Could you check a few things on this model? Use its own coordinates, in mm. Give positions to 0.01 mm unless a question says otherwise; leave off trailing zeros. Loops run counter-clockwise (first coordinate to the right, second up) from the corner with the lowest first, then second, coordinate; pieces in that order, holes last. Notation, with made-up numbers: (-34.5, 2) - (-24.5, 2) arc R31 ccw to (-24.5, 38) - close; hole circle Ø1 at (20.5, -39). An arc over 180 degrees is marked (long way). Write each question's results on one line, items separated by ' | '. Start each with the question number.
(1) Suppose I cut it at A-A (y = 0). Please give me the cut outline in (x, z) (3 decimals), and give its area (3 significant figures).
(2) Suppose I cut it at D-D (x = 18). Please give me the cut outline in (y, z) (3 decimals), and give its area (3 significant figures).
(3) Suppose I cut it at B-B (x = -9.5). Please give me the cut outline in (y, z) (3 decimals), and give its area (3 significant figures).
(4) Suppose I cut it at C-C (y = 4.5). Please give me the cut outline in (x, z) (3 decimals), and give its area (3 significant figures).
(5) I need wall thicknesses on line 1 (Y direction, x = 19.05, z = 0.6); line 2 (X direction, y = 9.5, z = 2.4); line 3 (Y direction, x = 0, z = 1.2). Which ranges of each line are inside material? Lowest first, please.
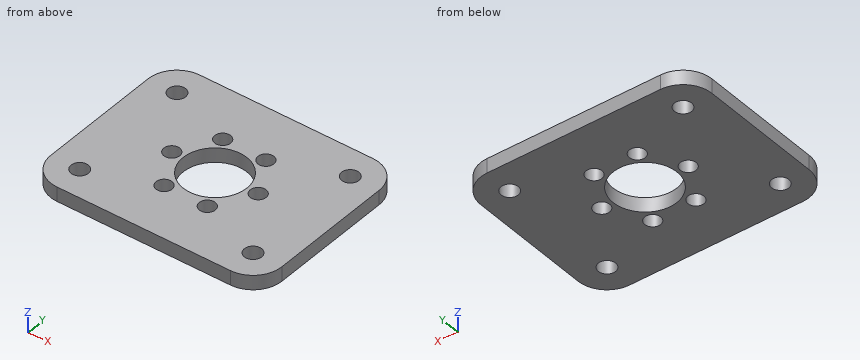
from build123d import *

# Parameters (mm, degrees)
SKETCH1_W           = 50.8
SKETCH1_H           = 40
SKETCH1_R           = 7
BOSS_EXTRUDE1_DEPTH = 3.175
FILLET1_R           = 6.35
SKETCH9_R           = 1.75
M3_THROUGH_DEPTH    = 4.175
SKETCH10_R          = 1.89865
CUT_EXTRUDE2_DEPTH  = 4.175


with BuildPart() as part:
    # Sketch1 → Boss-Extrude1 (new body)
    with BuildSketch(Plane.XY):
        Rectangle(SKETCH1_W, SKETCH1_H)
        Circle(SKETCH1_R, mode=Mode.SUBTRACT)
    extrude(amount=BOSS_EXTRUDE1_DEPTH)

    # Fillet1
    fillet1_edges = [part.edges().sort_by_distance(p)[0] for p in [
        (-25.4, 20, 1.5875),
        (25.4, 20, 1.5875),
        (25.4, -20, 1.5875),
        (-25.4, -20, 1.5875),
    ]]
    fillet(fillet1_edges, radius=FILLET1_R)

    # Sketch9 → M3-through (cut, through all)
    with BuildSketch(Plane.XY.offset(3.175)):
        with Locations((9.5, 0)):
            Circle(SKETCH9_R)
        with Locations((4.75, -8.227241336)):
            Circle(SKETCH9_R)
        with Locations((-4.75, -8.227241336)):
            Circle(SKETCH9_R)
        with Locations((-9.5, 0)):
            Circle(SKETCH9_R)
        with Locations((-4.75, 8.227241336)):
            Circle(SKETCH9_R)
        with Locations((4.75, 8.227241336)):
            Circle(SKETCH9_R)
    extrude(amount=-M3_THROUGH_DEPTH, mode=Mode.SUBTRACT)

    # Sketch10 → Cut-Extrude2 (cut, through all)
    with BuildSketch(Plane.XY.offset(3.175)):
        with Locations((19.05, -13.65)):
            Circle(SKETCH10_R)
        with Locations((19.05, 13.65)):
            Circle(SKETCH10_R)
        with Locations((-19.05, -13.65)):
            Circle(SKETCH10_R)
        with Locations((-19.05, 13.65)):
            Circle(SKETCH10_R)
    extrude(amount=-CUT_EXTRUDE2_DEPTH, mode=Mode.SUBTRACT)


solid = part.part
Output values:
1) outline: (-25.4, 0) - (-11.25, 0) - (-11.25, 3.175) - (-25.4, 3.175) - close; (-7.75, 0) - (-7, 0) - (-7, 3.175) - (-7.75, 3.175) - close; (7, 0) - (7.75, 0) - (7.75, 3.175) - (7, 3.175) - close; (11.25, 0) - (25.4, 0) - (25.4, 3.175) - (11.25, 3.175) - close | area: 94.6 mm2
2) outline: (-20, 0) - (-15.232, 0) - (-15.232, 3.175) - (-20, 3.175) - close; (-12.068, 0) - (12.068, 0) - (12.068, 3.175) - (-12.068, 3.175) - close; (15.232, 0) - (20, 0) - (20, 3.175) - (15.232, 3.175) - close | area: 107 mm2
3) outline: (-20, 0) - (-1.75, 0) - (-1.75, 3.175) - (-20, 3.175) - close; (1.75, 0) - (20, 0) - (20, 3.175) - (1.75, 3.175) - close | area: 116 mm2
4) outline: (-25.4, 0) - (-5.362, 0) - (-5.362, 3.175) - (-25.4, 3.175) - close; (5.362, 0) - (25.4, 0) - (25.4, 3.175) - (5.362, 3.175) - close | area: 127 mm2
5) line 1: -20 to -15.55, -11.75 to 11.75, 15.55 to 20 | line 2: -25.4 to -5.95, -3.55 to 3.55, 5.95 to 25.4 | line 3: -20 to -7, 7 to 20
